Here's how the part is built. I have some questions about the finished solid (model axes, mm). Round coordinates to 2 decimals unless told otherwise and drop trailing zeros. Write each loop counter-clockwise with the first axis right and the second up, starting at its lowest first coordinate (ties: lowest second). Pieces come first, ordered by that corner, then holes. Notation, with made-up numbers: (40.25, 38) -> (73.25, 38) arc R34 cw to (73.25, 69) -> close; hole circle Ø8 at (73, 25). An arc over 180 degrees is marked (long way). Answer as CSV lines item,"result".
```python
from build123d import *

# Parameters (mm, degrees)
PAD_DEPTH   = 0.8
FILLET_R    = 0.9
FILLET001_R = 0.75
FILLET002_R = 1.5


with BuildPart() as part:
    # Sketch → Pad (new body)
    with BuildSketch(Plane.XY):
        Polygon((-20.5, 12), (20.5, 12), (20.5, 1.5), (22.5, 1.5), (22.5, 9), (28.5, 9), (28.5, -9), (22.5, -9), (22.5, -1.5), (20.5, -1.5), (20.5, -12), (-20.5, -12), align=None)
    extrude(amount=PAD_DEPTH)

    # Fillet
    fillet_edges = [part.edges().sort_by_distance(p)[0] for p in [
        (22.5, -1.5, 0.4),
        (22.5, 1.5, 0.4),
        (20.5, 1.5, 0.4),
        (20.5, -1.5, 0.4),
    ]]
    fillet(fillet_edges, radius=FILLET_R)

    # Fillet001
    fillet001_edges = [part.edges().sort_by_distance(p)[0] for p in [
        (22.5, -9, 0.4),
        (28.5, -9, 0.4),
        (28.5, 9, 0.4),
        (22.5, 9, 0.4),
    ]]
    fillet(fillet001_edges, radius=FILLET001_R)

    # Fillet002
    fillet002_edges = [part.edges().sort_by_distance(p)[0] for p in [
        (20.5, -12, 0.4),
        (-20.5, -12, 0.4),
        (-20.5, 12, 0.4),
        (20.5, 12, 0.4),
    ]]
    fillet(fillet002_edges, radius=FILLET002_R)


solid = part.part
```
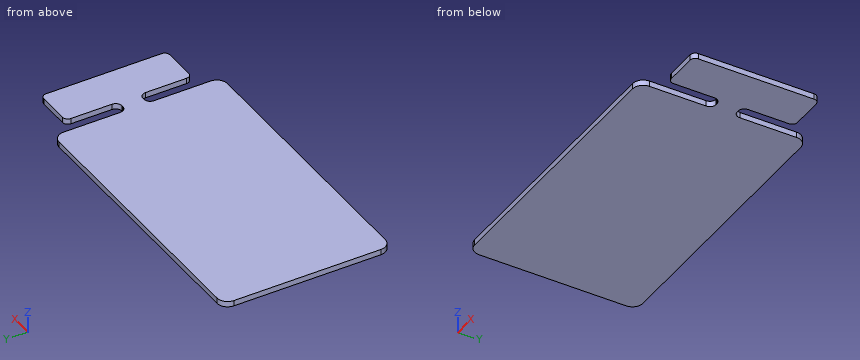
1. If I drill on line 1 (X direction, y = 4.5, z = 0.3); line 2 (X direction, y = 10, z = 0.45); line 3 (X direction, y = 8.75, z = 0.2), over which ranges is the centre line in solid material (lowest first)?
Numbers:
line 1,"x = -20.5 to 20.5, 22.5 to 28.5"
line 2,"x = -20.5 to 20.5"
line 3,"x = -20.5 to 20.5, 22.69 to 28.31"
2. Suppose I cut it at B-B on z = 0.6. Please give me the cut outline in (x, y), and give its area (3 significant figures).
Numbers:
outline,"(-20.5, -10.5) arc R1.5 ccw to (-19, -12) -> (19, -12) arc R1.5 ccw to (20.5, -10.5) -> (20.5, -2.4) arc R0.9 cw to (21.4, -1.5) -> (21.6, -1.5) arc R0.9 cw to (22.5, -2.4) -> (22.5, -8.25) arc R0.75 ccw to (23.25, -9) -> (27.75, -9) arc R0.75 ccw to (28.5, -8.25) -> (28.5, 8.25) arc R0.75 ccw to (27.75, 9) -> (23.25, 9) arc R0.75 ccw to (22.5, 8.25) -> (22.5, 2.4) arc R0.9 cw to (21.6, 1.5) -> (21.4, 1.5) arc R0.9 cw to (20.5, 2.4) -> (20.5, 10.5) arc R1.5 ccw to (19, 12) -> (-19, 12) arc R1.5 ccw to (-20.5, 10.5) -> close"
area,"1,100 mm^2"
3. Suppose I cut it at A-A on y = 5.25. Please give me the cut outline in (x, z), and give its area (3 significant figures).
Numbers:
outline,"(-20.5, 0) -> (20.5, 0) -> (20.5, 0.8) -> (-20.5, 0.8) -> close; (22.5, 0) -> (28.5, 0) -> (28.5, 0.8) -> (22.5, 0.8) -> close"
area,"37.6 mm^2"
